Part model, mm, in its own coordinate system. A direction names the side the tool comes from. Coordinates: 2 decimals unless noted, no trailing zeros. Loops run counter-clockwise (first coordinate to the right, second up) from the corner with the lowest first, then second, coordinate; pieces in that order, holes last. Notation, with made-up numbers: (0.5, 62.25) - (14.5, 62.25) arc R6 ccw to (14.5, 72.25) - close; hole circle Ø10 at (14, -33). An arc over 180 degrees is marked (long way). Use a Markdown table: item, result. Add a question column.
1) Drop flat-ended pins along their axis: P1, Ø1.5, axis at x = 37.5, y = 27, coming from the +Z side; P2, Ø8.5, axis at x = 39.5, y = 160, coming from the +Z side. Give the stop position or say it passes through.
2) Band-saw the part on C-C (y = 146.82). Give the cut face in (x, z), plus the area to 3 significant figures.
3) Band-saw the part on A-A (z = -34). Give the cut face in (x, y), plus the area to 3 significant figures.
4) Pull direction Z, two halves, no side cores. Call faces 1 (the face through (30.5, 112, -35)), 2 (the face through (30, 99, -60)), 3 (the face through (1, 100, 0)), 4 (the face through (1.48, 140.55, -28.47)): +Z half, -Z half, draft (parallel to the pull), parting line (faces both ways), or undercut.
5) Probe probe 1 along Z at (x, y) = (33, 111); probe 2 along Y at (x, z) = (32.5, -22.5); probe 3 along Y at (x, z) = (5.5, -33.5). List the from-to ranges inside material, lowest first. Write a range as [from, to].
6) Tool access for faces 5 (the face through (30, 0, -30)), 6 (the face through (57, 99, -28)): list every direction of +Z, -Z, +X, -X, +Y, -Y with a clear straight run to the whole face (end or side of a thin tool).
7) Band-saw the part on D-D (y = 70). Give the cut face in (x, z), plus the area to 3 significant figures.
8) Band-saw the part on B-B (x = 32.5). Give the cut face in (y, z), plus the area to 3 significant figures.
from build123d import *

# Parameters (mm, degrees)
SZKIC1_W                    = 60
SZKIC1_H                    = 60
DODANIE_WYCI_GNI_CIE1_DEPTH = 200
SKORUPA1_T                  = -3
SZKIC2_W                    = 5
SZKIC2_H                    = 5
SZKIC2_R                    = 1
DODANIE_WYCI_GNI_CIE5_DEPTH = 57
SZKIC3_W                    = 5
SZKIC3_H                    = 5
SZKIC3_R                    = 1
DODANIE_WYCI_GNI_CIE6_DEPTH = 57
SZKIC4_W                    = 5
SZKIC4_H                    = 5
SZKIC4_R                    = 1
DODANIE_WYCI_GNI_CIE7_DEPTH = 57
SZKIC5_W                    = 5
SZKIC5_H                    = 5
SZKIC5_R                    = 1
DODANIE_WYCI_GNI_CIE8_DEPTH = 57
SZKIC10_R                   = 10.3
WYTNIJ_WYCI_GNI_CIE3_DEPTH  = 3
SZKIC12_W                   = 45.55
SZKIC12_H                   = 7.6
DODANIE_WYCI_GNI_CIE9_DEPTH = 26.5
SZKIC13_R                   = 1.5
WYTNIJ_WYCI_GNI_CIE4_DEPTH  = 5
SZKIC15_R                   = 1.5
WYTNIJ_WYCI_GNI_CIE5_DEPTH  = 5
WYTNIJ_WYCI_GNI_CIE6_DEPTH  = 10
SZKIC17_W                   = 2
SZKIC17_H                   = 6
WYTNIJ_WYCI_GNI_CIE7_DEPTH  = 10


with BuildPart() as part:
    # Szkic1 → Dodanie-wyciągnięcie1 (new body)
    with BuildSketch(Plane(origin=(0, 0, 0), x_dir=(1, 0, 0), z_dir=(0, 1, 0))):
        with Locations((30, 30)):
            Rectangle(SZKIC1_W, SZKIC1_H)
    extrude(amount=DODANIE_WYCI_GNI_CIE1_DEPTH)

    # Skorupa1
    skorupa1_openings = [part.faces().sort_by_distance(p)[0] for p in [
        (30, 100, 0),
    ]]
    offset(amount=SKORUPA1_T, openings=skorupa1_openings, kind=Kind.INTERSECTION)

    # Szkic2 → Dodanie-wyciągnięcie5 (add)
    with BuildSketch(Plane.XY.offset(-57)):
        with Locations((5.5, 194.5)):
            Rectangle(SZKIC2_W, SZKIC2_H)
        with Locations(Location((5.5, 194.5, 0), (0, 0, 180))):
            Circle(SZKIC2_R, mode=Mode.SUBTRACT)
    extrude(amount=DODANIE_WYCI_GNI_CIE5_DEPTH)

    # Szkic3 → Dodanie-wyciągnięcie6 (add)
    with BuildSketch(Plane.XY.offset(-57)):
        with Locations((54.5, 194.5)):
            Rectangle(SZKIC3_W, SZKIC3_H)
        with Locations(Location((54.5, 194.5, 0), (0, 0, 180))):
            Circle(SZKIC3_R, mode=Mode.SUBTRACT)
    extrude(amount=DODANIE_WYCI_GNI_CIE6_DEPTH)

    # Szkic4 → Dodanie-wyciągnięcie7 (add)
    with BuildSketch(Plane.XY):
        with Locations((5.5, 5.5)):
            Rectangle(SZKIC4_W, SZKIC4_H)
        with Locations((5.5, 5.5)):
            Circle(SZKIC4_R, mode=Mode.SUBTRACT)
    extrude(amount=-DODANIE_WYCI_GNI_CIE7_DEPTH)

    # Szkic5 → Dodanie-wyciągnięcie8 (add)
    with BuildSketch(Plane.XY.offset(-57)):
        with Locations((54.5, 5.5)):
            Rectangle(SZKIC5_W, SZKIC5_H)
        with Locations(Location((54.5, 5.5, 0), (0, 0, 180))):
            Circle(SZKIC5_R, mode=Mode.SUBTRACT)
    extrude(amount=DODANIE_WYCI_GNI_CIE8_DEPTH)

    # Szkic10 → Wytnij-wyciągnięcie3 (cut)
    with BuildSketch(Plane.ZY):
        with Locations((-20.3, 146.82)):
            Circle(SZKIC10_R)
    extrude(amount=-WYTNIJ_WYCI_GNI_CIE3_DEPTH, mode=Mode.SUBTRACT)

    # Szkic12 → Dodanie-wyciągnięcie9 (add)
    with BuildSketch(Plane.ZY.offset(-57)):
        with Locations((-34.225, 160.62)):
            Rectangle(SZKIC12_W, SZKIC12_H)
        with Locations((-34.225, 112.02)):
            Rectangle(SZKIC12_W, SZKIC12_H)
    extrude(amount=DODANIE_WYCI_GNI_CIE9_DEPTH)

    # Szkic13 → Wytnij-wyciągnięcie4 (cut)
    with BuildSketch(Plane.ZY.offset(-30.5)):
        with Locations((-15.45, 162.42)):
            Circle(SZKIC13_R)
        with Locations((-25.1, 162.42)):
            Circle(SZKIC13_R)
    extrude(amount=-WYTNIJ_WYCI_GNI_CIE4_DEPTH, mode=Mode.SUBTRACT)

    # Szkic15 → Wytnij-wyciągnięcie5 (cut)
    with BuildSketch(Plane.ZY.offset(-30.5)):
        with Locations((-15.45, 111.22)):
            Circle(SZKIC15_R)
        with Locations((-25.1, 111.22)):
            Circle(SZKIC15_R)
    extrude(amount=-WYTNIJ_WYCI_GNI_CIE5_DEPTH, mode=Mode.SUBTRACT)

    # Szkic16 → Wytnij-wyciągnięcie6 (cut)
    with BuildSketch(Plane(origin=(0, 164.42, 0), x_dir=(1, 0, 0), z_dir=(0, 1, 0))):
        Polygon((57, 11.45), (57, 26.45), (48, 11.45), align=None)
    extrude(amount=-WYTNIJ_WYCI_GNI_CIE6_DEPTH, mode=Mode.SUBTRACT)

    # Szkic17 → Wytnij-wyciągnięcie7 (cut)
    with BuildSketch(Plane.ZY):
        with Locations((-20.3, 178.56)):
            Rectangle(SZKIC17_W, SZKIC17_H)
    extrude(amount=-WYTNIJ_WYCI_GNI_CIE7_DEPTH, mode=Mode.SUBTRACT)


solid = part.part
Answer block:
| question | item | result |
|---|---|---|
| 1 | P1 | z = -57 |
| 1 | P2 | z = -11.45 |
| 2 | outline | (0, -60) - (60, -60) - (60, 0) - (57, 0) - (57, -57) - (3, -57) - (3, -30.6) - (0, -30.6) - close; (0, -10) - (3, -10) - (3, 0) - (0, 0) - close |
| 2 | area | 460 mm2 |
| 3 | outline | (0, 0) - (60, 0) - (60, 200) - (0, 200) - close; hole (3, 8) - (8, 8) - (8, 3) - (52, 3) - (52, 8) - (57, 8) - (57, 108.22) - (30.5, 108.22) - (30.5, 115.82) - (57, 115.82) - (57, 156.82) - (30.5, 156.82) - (30.5, 164.42) - (57, 164.42) - (57, 192) - (52, 192) - (52, 197) - (8, 197) - (8, 192) - (3, 192) - close; hole circle Ø2 at (5.5, 5.5); hole circle Ø2 at (5.5, 194.5); hole circle Ø2 at (54.5, 5.5); hole circle Ø2 at (54.5, 194.5) |
| 3 | area | 2,010 mm2 |
| 4 | face 1 | draft |
| 4 | face 2 | -Z half |
| 4 | face 3 | +Z half |
| 4 | face 4 | undercut |
| 5 | probe 1 | [-60, -26.58], [-23.62, -16.93], [-13.97, -11.45] |
| 5 | probe 2 | [0, 3], [108.22, 115.82], [156.82, 164.42], [197, 200] |
| 5 | probe 3 | [0, 4.5], [6.5, 8], [192, 193.5], [195.5, 200] |
| 6 | face 5 | +Z, -Z, +X, -X, -Y |
| 6 | face 6 | +Z |
| 7 | outline | (0, -60) - (60, -60) - (60, 0) - (57, 0) - (57, -57) - (3, -57) - (3, 0) - (0, 0) - close |
| 7 | area | 522 mm2 |
| 8 | outline | (0, -60) - (200, -60) - (200, 0) - (197, 0) - (197, -57) - (164.42, -57) - (164.42, -11.45) - (156.82, -11.45) - (156.82, -57) - (115.82, -57) - (115.82, -11.45) - (108.22, -11.45) - (108.22, -57) - (3, -57) - (3, 0) - (0, 0) - close; hole circle Ø3 at (111.22, -25.1); hole circle Ø3 at (111.22, -15.45); hole circle Ø3 at (162.42, -25.1); hole circle Ø3 at (162.42, -15.45) |
| 8 | area | 1,610 mm2 |
